Part model, mm, in its own coordinate system. A direction names the side the tool comes from. Coordinates: 2 decimals unless noted, no trailing zeros. Loops run counter-clockwise (first coordinate to the right, second up) from the corner with the lowest first, then second, coordinate; pieces in that order, holes last. Notation, with made-up numbers: M 53,9 L 105,9 A7 cw 105,19 Z; hole C -17.75,33 d7. An arc over 180 degrees is marked long. Answer as CSV lines item,"result". Start each with the question number.
from build123d import *

# Parameters (mm, degrees)
SKETCH1_W               = 50
SKETCH1_H               = 50
BOSS_EXTRUDE1_DEPTH     = 15
SHELL1_T                = -3
CUT_EXTRUDE1_DEPTH      = 1
CUT_EXTRUDE1_DEPTH_BACK = 16
SKETCH5_W               = 7.5
SKETCH5_H               = 10
SKETCH5_H_2             = 12
CUT_EXTRUDE2_DEPTH      = 1
CUT_EXTRUDE2_DEPTH_BACK = 51
SKETCH6_W               = 12
SKETCH6_H               = 7.5
SKETCH6_W_2             = 10
CUT_EXTRUDE3_DEPTH      = 1
CUT_EXTRUDE3_DEPTH_BACK = 51


with BuildPart() as part:
    # Sketch1 → Boss-Extrude1 (new body)
    with BuildSketch(Plane.XY):
        Rectangle(SKETCH1_W, SKETCH1_H)
    extrude(amount=BOSS_EXTRUDE1_DEPTH)

    # Shell1
    shell1_openings = [part.faces().sort_by_distance(p)[0] for p in [
        (0, 0, 0),
    ]]
    offset(amount=SHELL1_T, openings=shell1_openings, kind=Kind.INTERSECTION)

    # Sketch2 → Cut-Extrude1 (cut, two sides)
    with BuildSketch(Plane(origin=(0, 0, 0), x_dir=(-1, 0, 0), z_dir=(0, 0, -1))) as cut_extrude1_sk:
        with BuildLine():
            Line((-2.15, 1.37113092), (-2.15, -1.37113092))
            ThreePointArc((-2.15, -1.37113092), (0, -2.55), (2.15, -1.37113092))
            Line((2.15, -1.37113092), (2.15, 1.37113092))
            ThreePointArc((2.15, 1.37113092), (0, 2.55), (-2.15, 1.37113092))
        make_face()
    extrude(amount=CUT_EXTRUDE1_DEPTH, mode=Mode.SUBTRACT)
    extrude(cut_extrude1_sk.sketch, amount=-CUT_EXTRUDE1_DEPTH_BACK, mode=Mode.SUBTRACT)

    # Sketch5 → Cut-Extrude2 (cut, two sides)
    with BuildSketch(Plane.ZY.offset(25)) as cut_extrude2_sk:
        with Locations((5.75, 15)):
            Rectangle(SKETCH5_W, SKETCH5_H)
        with Locations((5.75, 0)):
            Rectangle(SKETCH5_W, SKETCH5_H_2)
        with Locations((5.75, -15)):
            Rectangle(SKETCH5_W, SKETCH5_H)
    extrude(amount=CUT_EXTRUDE2_DEPTH, mode=Mode.SUBTRACT)
    extrude(cut_extrude2_sk.sketch, amount=-CUT_EXTRUDE2_DEPTH_BACK, mode=Mode.SUBTRACT)

    # Sketch6 → Cut-Extrude3 (cut, two sides)
    with BuildSketch(Plane.XZ.offset(25)) as cut_extrude3_sk:
        with Locations((0, 5.75)):
            Rectangle(SKETCH6_W, SKETCH6_H)
        with Locations((15, 5.75)):
            Rectangle(SKETCH6_W_2, SKETCH6_H)
        with Locations((-15, 5.75)):
            Rectangle(SKETCH6_W_2, SKETCH6_H)
    extrude(amount=CUT_EXTRUDE3_DEPTH, mode=Mode.SUBTRACT)
    extrude(cut_extrude3_sk.sketch, amount=-CUT_EXTRUDE3_DEPTH_BACK, mode=Mode.SUBTRACT)


solid = part.part
Q1. Slice it at C-C, the plane z = 11. Write the cut outline in (x, y).
Q2. Two-plate mould, pull along Z, no slides. Class faces 1 (the face through (-6, -24, 6)), 2 (the face through (-25, 0, 11)), 3 (the face through (-5, 0, 12)): +Z half, -Z half, draft (parallel to the pull), parting line (faces both ways), or undercut.
Q3. Tool access for faces 4 (the face through (0, 23, 2)), 5 (the face through (0, -25, 11)), 6 (the face through (23, 15, 9.5)), 7 (the face through (2.15, 0, 13)): list every direction of +Z, -Z, +X, -X, +Y, -Y with a clear straight run to the whole face (end or side of a thin tool).
Q4. Flat gauge pins, fed straight in: P1, Ø4, axis at y = 11, z = 6.5, coming from the -X side; P2, Ø3.5, axis at x = -2.5, z = 7, coming from the -Y side; P3, Ø2, axis at x = 7, y = -4.5, coming from the -Z side. Where does each tip first touch, or does it go through?
Q5. Slice it at A-A, the plane y = 13. Write the cut outline in (x, z).
Q6. Slice it at D-D, the plane x = 1. Write the cut outline in (y, z).
Q7. Wall check: L1, parallel to Y at x = 2, z = 11; L2, parallel to Z at x = 20.5, y = 21. Give the ranges that are in metal, low to high.
Solved:
1,outline,"M -25,-25 L 25,-25 L 25,25 L -25,25 Z; hole M -22,-22 L 22,-22 L 22,22 L -22,22 Z"
2,face 1,"undercut"
2,face 2,"draft"
2,face 3,"-Z half"
3,face 4,"+Y, -Y"
3,face 5,"+Z, -Z, +X, -X, -Y"
3,face 6,"+X, -X"
3,face 7,"+Z, -Z"
4,P1,"stops at x = -25"
4,P2,"passes through"
4,P3,"stops at z = 12"
5,outline,"M -25,0 L -22,0 L -22,2 L -25,2 Z; M -25,9.5 L -22,9.5 L -22,12 L 22,12 L 22,9.5 L 25,9.5 L 25,15 L -25,15 Z; M 22,0 L 25,0 L 25,2 L 22,2 Z"
6,outline,"M -25,0 L -22,0 L -22,2 L -25,2 Z; M -25,9.5 L -22,9.5 L -22,12 L -2.35,12 L -2.35,15 L -25,15 Z; M 2.35,12 L 22,12 L 22,9.5 L 25,9.5 L 25,15 L 2.35,15 Z; M 22,0 L 25,0 L 25,2 L 22,2 Z"
7,L1,"y = -25 to -22, 22 to 25"
7,L2,"z = 12 to 15"
